Print and shaded views of the part. All mm, measured from the part's lowest x, y and z. A direction names the side the tool comes from. Give positions to 0.01 mm unless a question says otherwise; leave off trailing zeros. Write each loop counter-clockwise with the first axis right and the second up, starting at its lowest first coordinate (ties: lowest second). Pieces come first, ordered by that corner, then holes. Notation, with made-up numbers: M -0.75,87 L 14.25,87 A7 cw 14.25,93 Z; hole C 24.5,63 d2. An arc over 180 degrees is marked long. One line per question, with ' | ' between items. Start each with the question number.
1. Cut at C-C, the plane z = 2.25. Write the cut outline in (x, y).
2. Pull direction X, two halves, no side cores. Call the marked faces 3, 4, 5 and 6: released by +X, released by -X, zero draft, split by the parting line, or undercut.
3. Which spindle directions (+Z, -Z, +X, -X, +Y, -Y) get a long thin tool onto all of the face, cutting with end or side? Do the marked faces 1 and 2. Say none if no direction does.
4. Wall check: L1, parallel to X at y = 1.7, z = 2.25; L2, parallel to Y at x = 2, z = 0.3; L3, parallel to Z at x = 2.05, y = 4.8. Give the ranges that are in metal, low to high.
5. Cut at B-B, the plane y = 3.5. Write the cut outline in (x, z), then the cut area to 3 significant figures.
6. Cut at A-A, the plane x = 2. Write the cut outline in (y, z), then the cut area to 4 significant figures.
7. Cut at D-D, the plane y = 0.85. Write the cut outline in (x, z), then the cut area to 3 significant figures.
8. Flat gauge pin, fed straight in: pin 1 (1.8 mm diameter, centred on x = 2, y = 3.5, fed in from +Z). Where does the tip first touch, or does it go through?
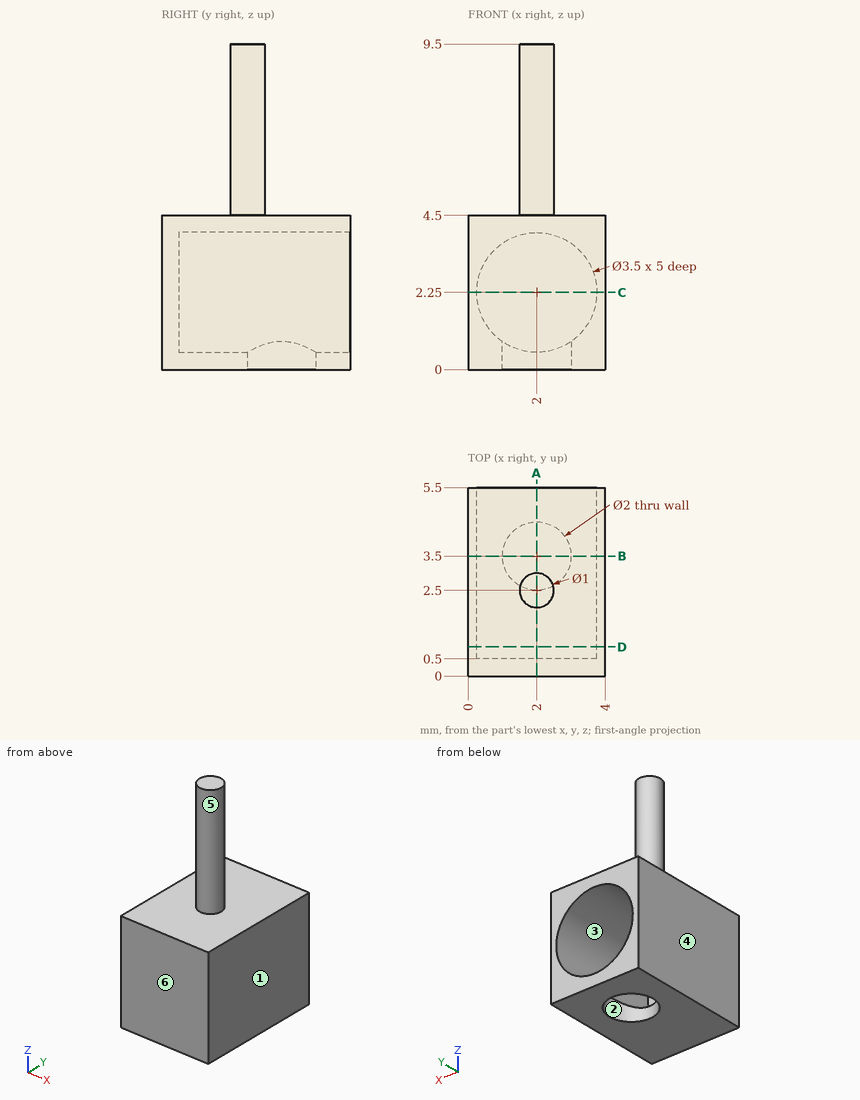
Here are the results:
1) outline: M 0,0 L 4,0 L 4,5.5 L 3.75,5.5 L 3.75,0.5 L 0.25,0.5 L 0.25,5.5 L 0,5.5 Z
2) face 3: undercut | face 4: released by -X | face 5: split by the parting line | face 6: zero draft
3) face 1: +Z, -Z, +X, +Y, -Y | face 2: -Z
4) L1: 0 to 0.25, 3.75 to 4 | L2: 0 to 2.5, 4.5 to 5.5 | L3: 0 to 0.5, 4 to 4.5
5) outline: M 0,0 L 1,0 L 1,0.81 A1.75 cw long 3,0.81 L 3,0 L 4,0 L 4,4.5 L 0,4.5 Z | area: 7.18 mm^2
6) outline: M 0,0 L 2.5,0 L 2.5,0.5 L 0.5,0.5 L 0.5,4 L 5.5,4 L 5.5,4.5 L 3,4.5 L 3,9.5 L 2,9.5 L 2,4.5 L 0,4.5 Z; M 4.5,0 L 5.5,0 L 5.5,0.5 L 4.5,0.5 Z | area: 11.25 mm^2
7) outline: M 0,0 L 4,0 L 4,4.5 L 0,4.5 Z; hole C 2,2.25 d3.5 | area: 8.38 mm^2
8) pin 1: z = 9.5
